Print and shaded views of the part. All mm, measured from the part's lowest x, y and z. A direction names the side the tool comes from. Give positions to 0.01 mm unless a question says otherwise; leave off trailing zeros. Order: outer loops, then holes, each group sorted by start corner. A loop starts at its lowest first (then second) coordinate and runs counter-clockwise, first axis right, second up. Notation, with made-up numbers: (-37.75, 34.25) - (-18.75, 34.25) arc R20 cw to (-18.75, 41.25) - close; hole circle Ø8 at (47.25, 63.5). An arc over 180 degrees is marked (long way). Answer in a Markdown table with one row per item.
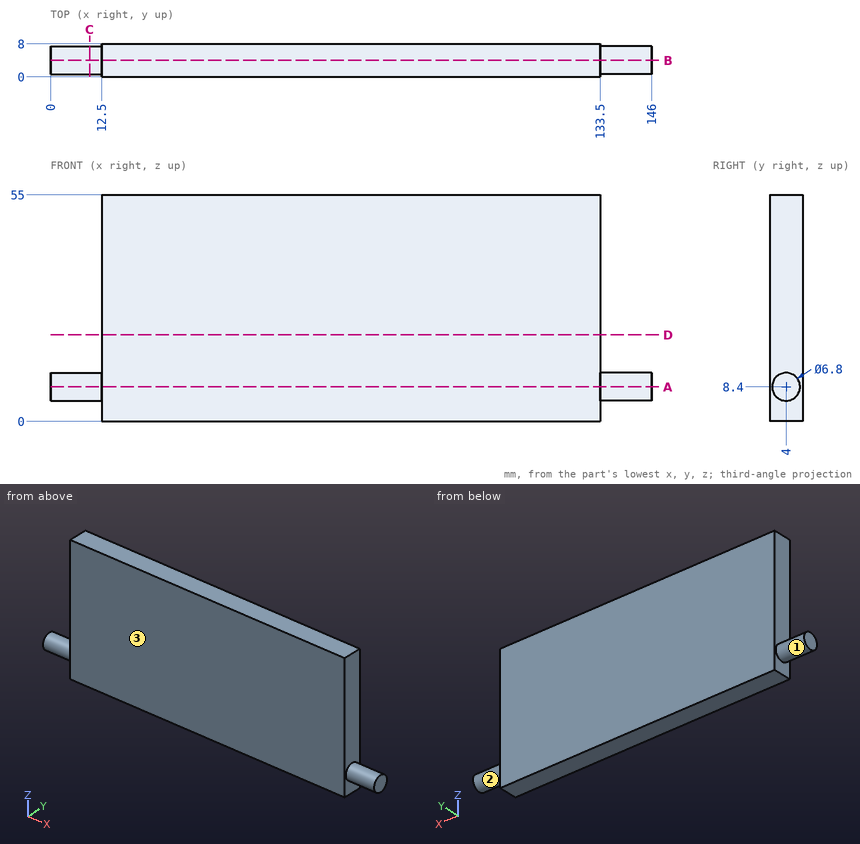
1. Cut at B-B on y = 4. Write the cut outline in (x, z).
Check result:
| item | result |
|---|---|
| outline | (0, 5) - (12.5, 5) - (12.5, 0) - (133.5, 0) - (133.5, 5) - (146, 5) - (146, 11.8) - (133.5, 11.8) - (133.5, 55) - (12.5, 55) - (12.5, 11.8) - (0, 11.8) - close |
2. Drop a flat-ended pin along its axis: P1, Ø4, axis at y = 3.5, z = 24, coming from the +X side. Give the stop position or say it passes through.
Check result:
| item | result |
|---|---|
| P1 | stops at x = 133.5 |
3. Cut at A-A on z = 8.4. Write the cut outline in (x, y), and give its area (3 significant figures).
Check result:
| item | result |
|---|---|
| outline | (0, 0.6) - (12.5, 0.6) - (12.5, 0) - (133.5, 0) - (133.5, 0.6) - (146, 0.6) - (146, 7.4) - (133.5, 7.4) - (133.5, 8) - (12.5, 8) - (12.5, 7.4) - (0, 7.4) - close |
| area | 1,140 mm² |
4. Cut at D-D on z = 21. Write the cut outline in (x, y), and give its area (3 significant figures).
Check result:
| item | result |
|---|---|
| outline | (12.5, 0) - (133.5, 0) - (133.5, 8) - (12.5, 8) - close |
| area | 968 mm² |
5. Cut at C-C on x = 9.5. Write the cut outline in (y, z).
Check result:
| item | result |
|---|---|
| outline | circle Ø6.8 at (4, 8.4) |
6. Which spindle directions (+Z, -Z, +X, -X, +Y, -Y) get a long thin tool onto all of the face, cutting with end or side? Do the marked faces 1, 2 and 3. Say none if no direction does.
Check result:
| item | result |
|---|---|
| face 1 | -X |
| face 2 | +X |
| face 3 | +Z, -Z, +X, -X, -Y |
7. Probe line 1 (X direction, y = 2.75, z = 42). List the from-to ranges inside material, lowest first.
Check result:
| item | result |
|---|---|
| line 1 | x = 12.5 to 133.5 |
